Geometry check sheet. Reference: the model listing, model coordinates, mm. Round coordinates to 2 decimals unless told otherwise and drop trailing zeros. Order: outer loops, then holes, each group sorted by start corner. A loop starts at its lowest first (then second) coordinate and runs counter-clockwise, first axis right, second up. Notation, with made-up numbers: (-6, 67) - (42, 67) arc R20 cw to (42, 85) - close; hole circle Ø11 at (42, 38). An arc over 180 degrees is marked (long way). Return JSON: item names as keys, results as strings. Group by question number.
Q1. Material ranges on line 1 along X through (y, z) = (0.55, 21.5); line 2 along Z through (x, y) = (-67.5, 0.9); line 3 along Z through (x, y) = (-38, 1.2), recorded low to high.
Q2. Sectioned sample at B-B, the plane z = -17. Record the cut outline in (x, y), then the cut area to 3 significant figures.
Q3. Gauge pin test, flat end, axial feed: pin 1 Ø0.6 at (y, z) = (0.5, 2.5) entering from +X. Record the tip position at first contact, or that the pin passes through.
Q4. Sectioned sample at A-A, the plane y = 1.1. Record the cut outline in (x, z), then the cut area to 3 significant figures.
Q5. Sectioned sample at C-C, the plane x = 47. Record the cut outline in (y, z), then the cut area to 3 significant figures.
Autodesk Inventor part; units mm, degrees
ref_plane "YZ Plane" through (0, 0, 0) normal (1, 0, 0) x (0, 1, 0)
ref_plane "XZ Plane" through (0, 0, 0) normal (0, 1, 0) x (-1, 0, 0)
ref_plane "XY Plane" through (0, 0, 0) normal (0, 0, 1) x (1, 0, 0)
sketch "Sketch1" plane through (0, 0, 0) normal (0, 1, 0) x (-1, 0, 0)
  line L0 (-75.5, -115.65) -> (-75.5, -62.65)
  line L1 (-65.5, -42.65) -> (-75.5, -62.65)
  line L2 (75.5, -115.65) -> (75.5, -62.65)
  line L3 (65.5, -42.65) -> (75.5, -62.65)
  line L4 (-75.5, 115.65) -> (-75.5, 42.15)
  line L5 (-65.5, 22.15) -> (-75.5, 42.15)
  line L6 (75.5, 115.65) -> (75.5, 42.15)
  line L7 (65.5, 22.15) -> (75.5, 42.15)
  line L8 (30.5, 135.65) -> (75.5, 115.65)
  line L9 (-30.5, 135.65) -> (-75.5, 115.65)
  line L10 (30.5, -135.65) -> (75.5, -115.65)
  line L11 (-30.5, -135.65) -> (-75.5, -115.65)
  line L12 (65.5, 22.15) -> (65.5, -42.65)
  line L13 (-65.5, -42.65) -> (-65.5, 22.15)
  line L14 (30.5, -135.65) -> (-30.5, -135.65)
  line L15 (30.5, 135.65) -> (-30.5, 135.65)
extrude "Extrusion1" add sketch "Sketch1" along normal blind 2
sketch "Sketch2" plane through (0, 2, 0) normal (0, 1, 0) x (1, 0, 0)
  line L0 (75.5, 62.65) -> (75.5, 115.65)
  line L1 (75.5, 115.65) -> (30.5, 135.65)
  line L2 (30.5, 135.65) -> (-30.5, 135.65)
  line L3 (-30.5, 135.65) -> (-75.5, 115.65)
  line L4 (-75.5, 115.65) -> (-75.5, 62.65)
  line L5 (-75.5, 62.65) -> (-65.5, 42.65)
  line L6 (-65.5, 42.65) -> (-65.5, -22.15)
  line L7 (-65.5, -22.15) -> (-75.5, -42.15)
  line L8 (-75.5, -115.65) -> (-30.5, -135.65)
  line L9 (-30.5, -135.65) -> (30.5, -135.65)
  line L10 (30.5, -135.65) -> (75.5, -115.65)
  line L11 (75.5, -115.65) -> (75.5, -42.15)
  line L12 (75.5, -42.15) -> (65.5, -22.15)
  line L13 (65.5, -22.15) -> (65.5, 42.65)
  line L14 (65.5, 42.65) -> (75.5, 62.65)
  line L15 (-75.5, -115.65) -> (75.5, -115.65)
  line L16 (-75.5, -42.15) -> (75.5, -42.15)
  line L17 (-75.5, 62.65) -> (75.5, 62.65)
  line L18 (-75.5, 115.65) -> (75.5, 115.65)
  line L19 (-75.5, 115.65) -> (-75.5, 105.65)
  line L20 (-75.5, 105.65) -> (75.5, 105.65)
  line L21 (75.5, 115.65) -> (75.5, 105.65)
  line L22 (-75.5, 62.65) -> (-75.5, 72.65)
  line L23 (-75.5, 72.65) -> (75.5, 72.65)
  line L24 (75.5, 62.65) -> (75.5, 72.65)
  line L25 (-75.5, -115.65) -> (-75.5, -105.65)
  line L26 (-75.5, -105.65) -> (75.5, -105.65)
  line L27 (75.5, -105.65) -> (75.5, -115.65)
  line L28 (-75.5, -62.65) -> (75.5, -62.65)
  line L29 (-65.5, 42.65) -> (-65.5, 120.0944)
  line L30 (65.5, 42.65) -> (65.5, 120.0944)
  line L31 (-65.5, -22.15) -> (-65.5, -120.0944)
  line L32 (65.5, -22.15) -> (65.5, -120.0944)
  line L33 (75.5, -62.65) -> (75.5, -72.65)
  line L34 (75.5, -72.65) -> (-75.5, -72.65)
  line L35 (-75.5, -62.65) -> (-75.5, -72.65)
  line L36 (-75.5, -42.15) -> (-75.5, -115.65)
  line L37 (65.5, -62.65) -> (40.6, -62.65)
  line L38 (40.6, -62.65) -> (40.6, -115.65)
  line L39 (40.6, -115.65) -> (50.6, -115.65)
  line L40 (50.6, -115.65) -> (50.6, -62.65)
  line L41 (50.6, -62.65) -> (40.6, -62.65)
  line L42 (-65.5, -62.65) -> (-40.6, -62.65)
  line L43 (-40.6, -62.65) -> (-40.6, -115.65)
  line L44 (-40.6, -115.65) -> (-50.6, -115.65)
  line L45 (-50.6, -115.65) -> (-50.6, -62.65)
  line L46 (-50.6, -62.65) -> (-40.6, -62.65)
  line L47 (-65.5, 115.65) -> (-40.6, 115.65)
  line L48 (-40.6, 115.65) -> (-40.6, 62.65)
  line L49 (-40.6, 62.65) -> (-50.6, 62.65)
  line L50 (-50.6, 62.65) -> (-50.6, 115.65)
  line L51 (-50.6, 115.65) -> (-40.6, 115.65)
  line L52 (65.5, 115.65) -> (40.6, 115.65)
  line L53 (40.6, 115.65) -> (40.6, 62.65)
  line L54 (40.6, 62.65) -> (50.6, 62.65)
  line L55 (50.6, 62.65) -> (50.6, 115.65)
  line L56 (50.6, 115.65) -> (40.6, 115.65)
  line L57 (-65.5, 12.65) -> (65.5, 12.65)
  line L58 (65.5, 12.65) -> (65.5, 22.65)
  line L59 (65.5, 22.65) -> (-65.5, 22.65)
  line L60 (-65.5, 22.65) -> (-65.5, 12.65)
  line L61 (0, 12.65) -> (0, -42.15)
  line L62 (-65.5, -42.15) -> (-65.5, 5.85)
  line L63 (-65.5, 5.85) -> (65.5, 5.85)
  line L64 (65.5, 5.85) -> (65.5, -42.15)
  line L65 (-65.5, -42.15) -> (-65.5, -40.15)
  line L66 (-65.5, -40.15) -> (65.5, -40.15)
  line L67 (65.5, -40.15) -> (65.5, -42.15)
  circle A0 centre (-70.5, 110.65) radius 1.2
  circle A1 centre (-70.5, 67.65) radius 1.2
  circle A2 centre (70.5, 110.65) radius 1.2
  circle A3 centre (70.5, 67.65) radius 1.2
  line L68 (-65.5, 115.65) -> (-24.1, 115.65)
  line L69 (65.5, 115.65) -> (24.1, 115.65)
  line L70 (-65.5, 72.65) -> (0, 72.65)
  line L71 (0, 22.65) -> (0, 17.65)
  circle A4 centre (0, 17.65) radius 1.2
  line L72 (-65.5, 22.65) -> (-60.5, 22.65)
  line L73 (-60.5, 22.65) -> (-60.5, 17.65)
  circle A5 centre (-60.5, 17.65) radius 1.2
  line L74 (65.5, 22.65) -> (60.5, 22.65)
  line L75 (60.5, 22.65) -> (60.5, 17.65)
  circle A6 centre (60.5, 17.65) radius 1.2
  line L76 (0, 5.85) -> (0, -17.15)
  line L77 (0, -17.15) -> (-32.15, -17.15)
  line L78 (0, -17.15) -> (32.15, -17.15)
  circle A7 centre (-32.15, -17.15) radius 1.2
  circle A8 centre (32.15, -17.15) radius 1.2
  line L79 (75.5, -42.15) -> (70.5, -42.15)
  circle A9 centre (70.5, -42.15) radius 1.2
  circle A10 centre (70.5, -67.65) radius 1.2
  circle A11 centre (70.5, -110.65) radius 1.2
  circle A12 centre (-70.5, -67.65) radius 1.2
  circle A13 centre (-70.5, -110.65) radius 1.2
  line L80 (-75.5, -42.15) -> (-70.5, -42.15)
  circle A14 centre (-70.5, -42.15) radius 1.2
  line L81 (0, -62.65) -> (0, -67.65)
  circle A15 centre (0, -67.65) radius 1.2
  line L82 (0, 115.65) -> (0, 110.65)
  circle A16 centre (0, 110.65) radius 1.2
  line L83 (-65.5, 72.65) -> (-24.1, 72.65)
  line L84 (-24.1, 72.65) -> (-24.1, 67.65)
  line L85 (65.5, 72.65) -> (24.1, 72.65)
  line L86 (24.1, 72.65) -> (24.1, 67.65)
  circle A17 centre (-24.1, 67.65) radius 1.2
  circle A18 centre (24.1, 67.65) radius 1.2
  line L87 (-65.5, -105.65) -> (-24.1, -105.65)
  line L88 (-24.1, -105.65) -> (-24.1, -110.65)
  line L89 (65.5, -105.65) -> (24.1, -105.65)
  line L90 (24.1, -105.65) -> (24.1, -110.65)
  circle A19 centre (-24.1, -110.65) radius 1.2
  circle A20 centre (24.1, -110.65) radius 1.2
  line L91 (-50.6, -62.65) -> (-50.6, -89.15)
  line L92 (-50.6, -89.15) -> (-45.6, -89.15)
  line L93 (40.6, -62.65) -> (40.6, -89.15)
  line L94 (40.6, -89.15) -> (45.6, -89.15)
  line L95 (40.6, 115.65) -> (40.6, 89.15)
  line L96 (40.6, 89.15) -> (45.6, 89.15)
  line L97 (-50.6, 115.65) -> (-50.6, 89.15)
  line L98 (-50.6, 89.15) -> (-45.6, 89.15)
  circle A21 centre (-45.6, 89.15) radius 1.2
  circle A22 centre (45.6, 89.15) radius 1.2
  circle A23 centre (45.6, -89.15) radius 1.2
  circle A24 centre (-45.6, -89.15) radius 1.2
  point P0 (0, 0)
  dimension "d26" = 10
  dimension "d27" = 10
  dimension "d28" = 10
  dimension "d29" = 53
  dimension "d30" = 10
  dimension "d31" = 24.9
  dimension "d32" = 53
  dimension "d33" = 10
  dimension "d35" = 24.9
  dimension "d36" = 10
  dimension "d37" = 53
  dimension "d38" = 24.9
  dimension "d39" = 53
  dimension "d40" = 10
  dimension "d41" = 53
  dimension "d42" = 24.9
  dimension "d43" = 53
  dimension "d44" = 10
  dimension "d45" = 53
  dimension "d47" = 131
  dimension "d48" = 10
  dimension "d49" = 131
  dimension "d50" = 54.8
  dimension "d51" = 48
  dimension "d52" = 131
  dimension "d53" = 2
  dimension "d54" = 131
  dimension "d68" = 5
  dimension "d70" = 5
  dimension "d71" = 5
  dimension "d73" = 5
  dimension "d74" = 5
  dimension "d76" = 23
  dimension "d77" = 32.15
  dimension "d78" = 32.15
  dimension "d86" = 5
  dimension "d88" = 5
  dimension "d90" = 5
  dimension "d92" = 41.4
  dimension "d93" = 5
  dimension "d94" = 41.4
  dimension "d98" = 41.4
  dimension "d99" = 5
  dimension "d100" = 41.4
  dimension "d101" = 5
  dimension "d104" = 26.5
  dimension "d105" = 5
  dimension "d106" = 26.5
  dimension "d107" = 5
  dimension "d108" = 26.5
  dimension "d109" = 5
  dimension "d110" = 26.5
  dimension "d111" = 5
sketch "Sketch3" plane through (0, 2, 0) normal (0, 1, 0) x (1, 0, 0)
  line L0 (75.5, 62.65) -> (75.5, 115.65)
  line L1 (75.5, 115.65) -> (30.5, 135.65)
  line L2 (30.5, 135.65) -> (-30.5, 135.65)
  line L3 (-30.5, 135.65) -> (-75.5, 115.65)
  line L4 (-75.5, 115.65) -> (-75.5, 62.65)
  line L5 (-75.5, 62.65) -> (-65.5, 42.65)
  line L6 (-65.5, 42.65) -> (-65.5, -22.15)
  line L7 (-65.5, -22.15) -> (-75.5, -42.15)
  line L8 (-75.5, -42.15) -> (-75.5, -115.65)
  line L9 (-75.5, -115.65) -> (-30.5, -135.65)
  line L10 (-30.5, -135.65) -> (30.5, -135.65)
  line L11 (30.5, -135.65) -> (75.5, -115.65)
  line L12 (75.5, -115.65) -> (75.5, -42.15)
  line L13 (75.5, -42.15) -> (65.5, -22.15)
  line L14 (65.5, -22.15) -> (65.5, 42.65)
  line L15 (65.5, 42.65) -> (75.5, 62.65)
  point P0 (0, 0)
  dimension "d116" = 271.3
  dimension "d117" = 151
  dimension "d118" = 64.8
  dimension "d119" = 20
properties part number "podvozek_+_prametry"
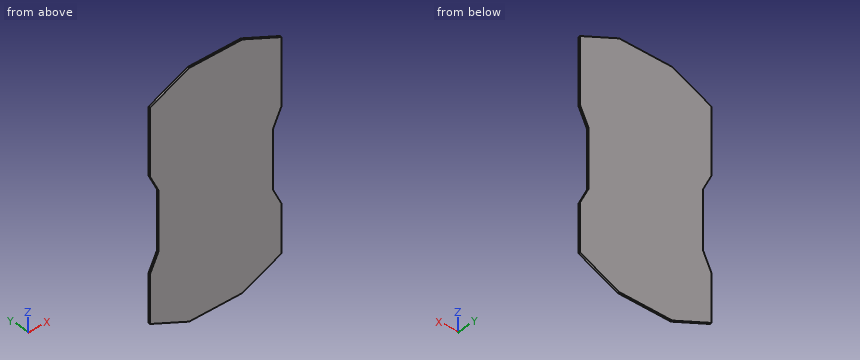
Reply:
{
 "1": {"line 1": "-65.5 to 65.5", "line 2": "-119.21 to -46.65, 26.15 to 119.21", "line 3": "-132.32 to 132.32"},
 "2": {"outline": "(-65.5, 0) - (65.5, 0) - (65.5, 2) - (-65.5, 2) - close", "area": "262 mm^2"},
 "3": {"pin 1": "x = 65.5"},
 "4": {"outline": "(-75.5, -115.65) - (-30.5, -135.65) - (30.5, -135.65) - (75.5, -115.65) - (75.5, -62.65) - (65.5, -42.65) - (65.5, 22.15) - (75.5, 42.15) - (75.5, 115.65) - (30.5, 135.65) - (-30.5, 135.65) - (-75.5, 115.65) - (-75.5, 42.15) - (-65.5, 22.15) - (-65.5, -42.65) - (-75.5, -62.65) - close", "area": "37,500 mm^2"},
 "5": {"outline": "(0, -128.32) - (2, -128.32) - (2, 128.32) - (0, 128.32) - close", "area": "513 mm^2"}
}
